```python
from build123d import *

# Parameters (mm, degrees)
SKETCH1_W                = 70
SKETCH1_H                = 45
BOSS_EXTRUDE1_DEPTH      = 6
CUT_EXTRUDE1_REACH       = 410.214
SKETCH4_R                = 1.5
SKETCH5_W                = 4
SKETCH5_H                = 45
BOSS_EXTRUDE2_DEPTH      = 138.11
CUT_EXTRUDE2_REACH       = 393.806
SKETCH6_R                = 3
FILLET1_R                = 25
BOSS_EXTRUDE3_DEPTH      = 1
BOSS_EXTRUDE3_DEPTH_BACK = 1


with BuildPart() as part:
    # Sketch1 → Boss-Extrude1 (new body)
    with BuildSketch(Plane(origin=(148.74203414, 0, 254.057769676), x_dir=(1, 0, 0), z_dir=(0, -1, 0))):
        with Locations((13.131189711, 80.994934751)):
            Rectangle(SKETCH1_W, SKETCH1_H)
    extrude(amount=-BOSS_EXTRUDE1_DEPTH)

    # Sketch4 → Cut-Extrude1 (cut, up to next)
    with BuildSketch(Plane(origin=(0, 6, 0), x_dir=(-1, 0, 0), z_dir=(0, 1, 0)), mode=Mode.PRIVATE) as cut_extrude1_sk1:
        with Locations(Location((-188.87322385, 320.552704426, 0), (0, 0, 90))):
            Circle(SKETCH4_R)
    cut_extrude1_tool1 = extrude(cut_extrude1_sk1.sketch, amount=-CUT_EXTRUDE1_REACH, mode=Mode.PRIVATE) & part.part
    # Sketch4 → Cut-Extrude1 (cut, up to next)
    with BuildSketch(Plane(origin=(0, 6, 0), x_dir=(-1, 0, 0), z_dir=(0, 1, 0)), mode=Mode.PRIVATE) as cut_extrude1_sk2:
        with Locations(Location((-188.87322385, 349.552704426, 0), (0, 0, 90))):
            Circle(SKETCH4_R)
    cut_extrude1_tool2 = extrude(cut_extrude1_sk2.sketch, amount=-CUT_EXTRUDE1_REACH, mode=Mode.PRIVATE) & part.part
    # Sketch4 → Cut-Extrude1 (cut, up to next)
    with BuildSketch(Plane(origin=(0, 6, 0), x_dir=(-1, 0, 0), z_dir=(0, 1, 0)), mode=Mode.PRIVATE) as cut_extrude1_sk3:
        with Locations(Location((-134.87322385, 320.552704426, 0), (0, 0, 90))):
            Circle(SKETCH4_R)
    cut_extrude1_tool3 = extrude(cut_extrude1_sk3.sketch, amount=-CUT_EXTRUDE1_REACH, mode=Mode.PRIVATE) & part.part
    # Sketch4 → Cut-Extrude1 (cut, up to next)
    with BuildSketch(Plane(origin=(0, 6, 0), x_dir=(-1, 0, 0), z_dir=(0, 1, 0)), mode=Mode.PRIVATE) as cut_extrude1_sk4:
        with Locations(Location((-134.87322385, 349.552704426, 0), (0, 0, 90))):
            Circle(SKETCH4_R)
    cut_extrude1_tool4 = extrude(cut_extrude1_sk4.sketch, amount=-CUT_EXTRUDE1_REACH, mode=Mode.PRIVATE) & part.part
    add(cut_extrude1_tool1.solids().sort_by_distance((188.873224, 6, 320.552704))[0], mode=Mode.SUBTRACT)
    add(cut_extrude1_tool2.solids().sort_by_distance((188.873224, 6, 349.552704))[0], mode=Mode.SUBTRACT)
    add(cut_extrude1_tool3.solids().sort_by_distance((134.873224, 6, 320.552704))[0], mode=Mode.SUBTRACT)
    add(cut_extrude1_tool4.solids().sort_by_distance((134.873224, 6, 349.552704))[0], mode=Mode.SUBTRACT)

    # Sketch5 → Boss-Extrude2 (add)
    with BuildSketch(Plane(origin=(0, 6, 0), x_dir=(-1, 0, 0), z_dir=(0, -1, 0))):
        with Locations((-128.87322385, -335.052704426)):
            Rectangle(SKETCH5_W, SKETCH5_H)
    boss_extrude2 = extrude(amount=-BOSS_EXTRUDE2_DEPTH)

    # Sketch6 → Cut-Extrude2 (cut, up to next)
    with BuildSketch(Plane.ZY.offset(-126.87322385), mode=Mode.PRIVATE) as cut_extrude2_sk1:
        with Locations((335.052704426, 137.11)):
            Circle(SKETCH6_R)
    cut_extrude2_tool1 = extrude(cut_extrude2_sk1.sketch, amount=-CUT_EXTRUDE2_REACH, mode=Mode.PRIVATE) & part.part
    # Sketch6 → Cut-Extrude2 (cut, up to next)
    with BuildSketch(Plane.ZY.offset(-126.87322385), mode=Mode.PRIVATE) as cut_extrude2_sk2:
        with Locations((335.052704426, 117.11)):
            Circle(SKETCH6_R)
    cut_extrude2_tool2 = extrude(cut_extrude2_sk2.sketch, amount=-CUT_EXTRUDE2_REACH, mode=Mode.PRIVATE) & part.part
    cut_extrude2_1 = cut_extrude2_tool1.solids().sort_by_distance((126.873224, 137.11, 335.052704))[0]
    add(cut_extrude2_1, mode=Mode.SUBTRACT)
    cut_extrude2_2 = cut_extrude2_tool2.solids().sort_by_distance((126.873224, 117.11, 335.052704))[0]
    add(cut_extrude2_2, mode=Mode.SUBTRACT)
    cut_extrude2 = cut_extrude2_1 + cut_extrude2_2  # Cut-Extrude2 as one shape, for the pattern or mirror that repeats it

    # Mirror1: Boss-Extrude2, Cut-Extrude2 across plane
    add(boss_extrude2.mirror(Plane(origin=(161.87322385, 0, 0), x_dir=(0, 0, 1), z_dir=(1, 0, 0))))
    add(cut_extrude2.mirror(Plane(origin=(161.87322385, 0, 0), x_dir=(0, 0, 1), z_dir=(1, 0, 0))), mode=Mode.SUBTRACT)

    # Fillet1
    # the kernel refuses this fillet: 25 mm, written as the material it takes off along each edge
    with BuildSketch(Plane(origin=(259.37322385, 144.11, 312.552704426), x_dir=(0, 0, 1), z_dir=(-1, 0, 0)), Plane(origin=(193.37322385, 144.11, 357.552704426), x_dir=(0, -1, 0), z_dir=(-1, 0, 0))) as fillet1_piece_1:
        with BuildLine():
            CenterArc((FILLET1_R, -FILLET1_R), FILLET1_R, 90, 90)
            Line((0, -FILLET1_R), (0, 0))
            Line((0, 0), (FILLET1_R, 0))
        make_face()
    extrude(amount=129, mode=Mode.SUBTRACT)
    with BuildSketch(Plane(origin=(130.37322385, 144.11, 357.552704426), x_dir=(0, -1, 0), z_dir=(1, 0, 0)), Plane(origin=(64.37322385, 144.11, 312.552704426), x_dir=(0, 0, 1), z_dir=(1, 0, 0))) as fillet1_piece_2:
        with BuildLine():
            CenterArc((FILLET1_R, FILLET1_R), FILLET1_R, 180, 90)
            Line((0, FILLET1_R), (0, 0))
            Line((0, 0), (FILLET1_R, 0))
        make_face()
    extrude(amount=129, mode=Mode.SUBTRACT)

    # Sketch8 → Boss-Extrude3 (add, two sides: drawn at the far end of the back side and taken through both)
    with BuildSketch(Plane(origin=(0, 0, 335.052704426), x_dir=(-1, 0, 0), z_dir=(0, 0, -1)).offset(-BOSS_EXTRUDE3_DEPTH_BACK)):
        Polygon((-192.87322385, 6), (-192.87322385, 26), (-179.87322385, 6), align=None)
        Polygon((-130.87322385, 26), (-143.87322385, 6), (-130.87322385, 6), align=None)
    extrude(amount=BOSS_EXTRUDE3_DEPTH + BOSS_EXTRUDE3_DEPTH_BACK)


solid = part.part
```
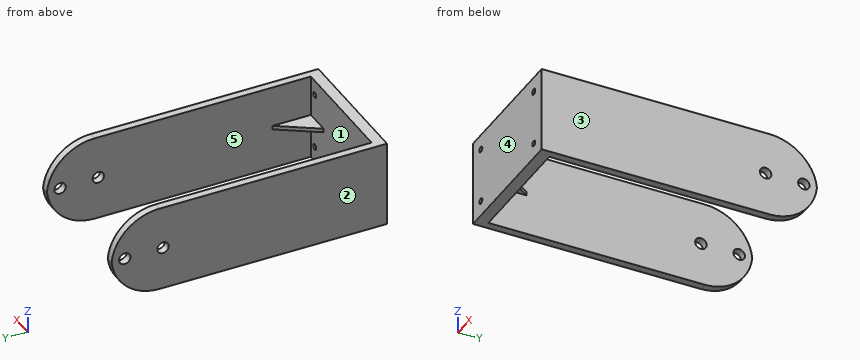
Build history of the part. All positions in model axes, mm. Face numbers are marked on the shaded views. A direction names the side the tool comes from. Give positions to 0.01 mm unless a question says otherwise; leave off trailing zeros. Loops run counter-clockwise (first coordinate to the right, second up) from the corner with the lowest first, then second, coordinate; pieces in that order, holes last. Notation, with made-up numbers: (-15.5, 41) -> (22.5, 41) arc R24 ccw to (22.5, 52) -> close; hole circle Ø1 at (45.5, -28.75). An arc over 180 degrees is marked (long way). One line per question, with ' | ' between items.
Q1. Cut at A-A, the plane y = 117.11. Write the cut outline in (x, z), plus the area to 3 significant figures.
Filled sheet:
outline: (126.87, 312.55) -> (130.87, 312.55) -> (130.87, 332.05) -> (126.87, 332.05) -> close; (126.87, 338.05) -> (130.87, 338.05) -> (130.87, 357.55) -> (126.87, 357.55) -> close; (192.87, 312.55) -> (196.87, 312.55) -> (196.87, 332.05) -> (192.87, 332.05) -> close; (192.87, 338.05) -> (196.87, 338.05) -> (196.87, 357.55) -> (192.87, 357.55) -> close | area: 312 mm²
Q2. Drill centre lines: line 1 along X through (y, z) = (117, 330.5); line 2 along Z through (x, y) = (128, 117); line 3 along Y through (x, z) = (192, 343.5). Where is each one in solid material? Low to high. Write a range as [from, to].
Filled sheet:
line 1: x = [126.87, 130.87], [192.87, 196.87] | line 2: z = [312.55, 332.05], [338.05, 357.55] | line 3: y = [0, 6]
Q3. Cut at C-C, the plane z = 320.5. Write the cut outline in (x, y), plus the area to 3 significant figures.
Filled sheet:
outline: (126.87, 0) -> (133.37, 0) -> (133.37, 6) -> (130.87, 6) -> (130.87, 137.39) -> (126.87, 137.39) -> close; (136.37, 0) -> (187.37, 0) -> (187.37, 6) -> (136.37, 6) -> close; (190.37, 0) -> (196.87, 0) -> (196.87, 137.39) -> (192.87, 137.39) -> (192.87, 6) -> (190.37, 6) -> close | area: 1,440 mm²
Q4. Pull direction X, two halves, no side cores. Call the marked faces 3, 4 and 5: pulls with the +X half, pulls with the -X half, needs draft (parallel to the pull), parting line crosses it, or undercut.
Filled sheet:
face 3: pulls with the +X half | face 4: needs draft | face 5: undercut
Q5. Tool access for the marked faces 1 and 2: list every direction of +Z, -Z, +X, -X, +Y, -Y with a clear straight run to the whole face (end or side of a thin tool).
Filled sheet:
face 1: +Y | face 2: +Z, -Z, -X, +Y, -Y
Q6. Cut at D-D, the plane z = 353. Write the cut outline in (x, y), plus the area to 3 significant figures.
Filled sheet:
outline: (126.87, 0) -> (196.87, 0) -> (196.87, 133.49) -> (192.87, 133.49) -> (192.87, 6) -> (130.87, 6) -> (130.87, 133.49) -> (126.87, 133.49) -> close | area: 1,440 mm²
Q7. Drop flat-ended pins along their axis: pin 1 (8 mm diameter, centred on x = 135.5, z = 341.5, fed in from -Y); pin 2 (13.5 mm diameter, centred on x = 150.5, z = 332.5, fed in from +Y); pin 3 (4 mm diameter, centred on x = 135, y = 20.5, fed in from +Z); pin 4 (14.5 mm diameter, centred on x = 140.5, y = 15, fed in from -Z). Give the stop position or say it passes through.
Filled sheet:
pin 1: stops at y = 0 | pin 2: stops at y = 6 | pin 3: stops at z = 336.05 | pin 4: stops at z = 334.05
Q8. Cut at B-B, the plane y = 62. Write the cut outline in (x, z), plus the area to 3 significant figures.
Filled sheet:
outline: (126.87, 312.55) -> (130.87, 312.55) -> (130.87, 357.55) -> (126.87, 357.55) -> close; (192.87, 312.55) -> (196.87, 312.55) -> (196.87, 357.55) -> (192.87, 357.55) -> close | area: 360 mm²
